```python
from build123d import *

# Parameters (mm, degrees)
F0_R     = 2.179644
F0_R_2   = 5.495
F0_R_3   = 1.811627
F0_R_4   = 2.717522
F1_DEPTH = 3


with BuildPart() as f1:
    # F0 (on Front) → F1 (new body)
    with BuildSketch(Plane.XZ):
        with BuildLine():
            ThreePointArc((4.748624, -43.868074), (19.905522, -31.458489), (38.356329, -38.03854))
            ThreePointArc((38.356329, -38.03854), (48.781106, -31.139926), (36.287612, -31.563568))
            ThreePointArc((36.287612, -31.563568), (34.479775, -16.939453), (26.872979, -4.319244))
            ThreePointArc((26.872979, -4.319244), (26.851679, 10.968683), (15.96134, 21.69816))
            ThreePointArc((15.96134, 21.69816), (22.323636, 32.655587), (20.63084, 45.212594))
            Line((20.63084, 45.212594), (46.282084, 75.748279))
            ThreePointArc((46.282084, 75.748279), (45.843056, 85.044031), (36.784028, 82.913828))
            ThreePointArc((36.784028, 82.913828), (23.791047, 69.810118), (12.145666, 55.495445))
            ThreePointArc((12.145666, 55.495445), (-7.14242, 61.665744), (-26.03866, 54.383233))
            ThreePointArc((-26.03866, 54.383233), (-44.027199, 51.327224), (-32.686998, 37.03294))
            ThreePointArc((-32.686998, 37.03294), (-31.643455, 28.376793), (-26.03866, 21.69816))
            ThreePointArc((-26.03866, 21.69816), (-36.080562, 10.571243), (-37.789793, -4.319244))
            ThreePointArc((-37.789793, -4.319244), (-47.116357, -23.066533), (-44.720202, -43.868074))
            ThreePointArc((-44.720202, -43.868074), (-26.129955, -31.677407), (-7.539708, -43.868074))
            ThreePointArc((-7.539708, -43.868074), (-1.395542, -49.586683), (4.748624, -43.868074))
        make_face()
        with Locations((-39.195588, -22.667399)):
            Circle(F0_R, mode=Mode.SUBTRACT)
        with BuildLine():
            ThreePointArc((2.764325, -43.460141), (-1.413553, -47.586646), (-5.555543, -43.424121))
            ThreePointArc((-5.555543, -43.424121), (-23.64801, -29.816144), (-44.305303, -39.078469))
            ThreePointArc((-44.305303, -39.078469), (-45.548112, -32.328702), (-45.443616, -25.466268))
            ThreePointArc((-45.443616, -25.466268), (-32.535702, -24.254044), (-43.510487, -17.352027))
            ThreePointArc((-43.510487, -17.352027), (-40.221713, -10.719441), (-35.605799, -4.931473))
            ThreePointArc((-35.605799, -4.931473), (-33.578613, 11.124985), (-21.324643, 21.696624))
            ThreePointArc((-21.324643, 21.696624), (-23.830093, 22.711263), (-26.078436, 24.211837))
            Line((-26.078436, 24.211837), (-13.440696, 31.617877))
            ThreePointArc((-13.440696, 31.617877), (-6.255235, 27.617264), (0.930225, 31.617877))
            Line((0.930225, 31.617877), (15.984657, 24.496045))
            ThreePointArc((15.984657, 24.496045), (13.79085, 22.50908), (11.294313, 20.919072))
            ThreePointArc((11.294313, 20.919072), (24.421465, 11.452539), (24.483739, -4.73182))
            ThreePointArc((24.483739, -4.73182), (29.09938, -10.414096), (32.365767, -16.96567))
            ThreePointArc((32.365767, -16.96567), (21.262061, -22.860799), (33.814338, -22.164239))
            ThreePointArc((33.814338, -22.164239), (34.375369, -26.760579), (34.29513, -31.390337))
            ThreePointArc((34.29513, -31.390337), (34.279314, -31.754857), (34.29513, -32.119377))
            ThreePointArc((34.29513, -32.119377), (15.892899, -30.458566), (2.764325, -43.460141))
        make_face(mode=Mode.SUBTRACT)
        with Locations((42.594204, -33.116606)):
            Circle(F0_R_2, mode=Mode.SUBTRACT)
        with Locations((27.461662, -21.133294)):
            Circle(F0_R_3, mode=Mode.SUBTRACT)
        with BuildLine():
            ThreePointArc((-29.585752, 40.232415), (-42.395978, 49.904419), (-26.407067, 51.320147))
            ThreePointArc((-26.407067, 51.320147), (-17.597387, 57.321958), (-7.197797, 59.663057))
            Line((-7.197797, 59.663057), (-7.403995, 44.445188))
            ThreePointArc((-7.403995, 44.445188), (-13.167698, 40.936028), (-14.526525, 34.326333))
            Line((-14.526525, 34.326333), (-28.093472, 26.283829))
            ThreePointArc((-28.093472, 26.283829), (-30.829773, 33.045206), (-29.585752, 40.232415))
        make_face(mode=Mode.SUBTRACT)
        with Locations((-6.255235, 36.070436)):
            Circle(F0_R_4, mode=Mode.SUBTRACT)
        with BuildLine():
            Line((44.843853, 77.145583), (18.220686, 45.452904))
            ThreePointArc((18.220686, 45.452904), (20.692534, 36.023365), (17.751182, 26.729566))
            Line((17.751182, 26.729566), (1.985629, 34.18781))
            ThreePointArc((1.985629, 34.18781), (0.697801, 40.877869), (-5.106476, 44.445188))
            Line((-5.106476, 44.445188), (-5.106476, 59.655479))
            ThreePointArc((-5.106476, 59.655479), (4.312025, 57.645012), (12.521453, 52.609595))
            ThreePointArc((12.521453, 52.609595), (24.714277, 67.842383), (38.436119, 81.713713))
            ThreePointArc((38.436119, 81.713713), (44.55039, 83.512084), (44.843853, 77.145583))
        make_face(mode=Mode.SUBTRACT)
    extrude(amount=F1_DEPTH)


solid = f1.part
```
Part model, mm, in its own coordinate system. Coordinates: 2 decimals unless noted, no trailing zeros. Order: outer loops, then holes, each group sorted by start corner. A loop starts at its lowest first (then second) coordinate and runs counter-clockwise, first axis right, second up. Notation, with made-up numbers: (-40, -34.75) - (9, -34.75) arc R14 cw to (9, -21.75) - close; hole circle Ø8 at (81, -36.5). An arc over 180 degrees is marked (long way). Return JSON: item names as keys, results as strings. Group by question number.
Item 1: Cut at D-D (y = -1.65). State how many separate pieces and enclosed holes the cut face has, plus the area to 3 significant figures.
Item 2: Cut at B-B (x = -17). List the corners of the cut face in (y, z).
Item 3: Pin check, flat tips, straight feed: pin 1 (6.5 mm diameter, centred on x = -6.26, z = 36.07, fed in from -Y); pin 2 (1 mm diameter, centred on y = -1, z = 27, fed in from -X); pin 3 (1 mm diameter, centred on y = -1.5, z = 23, fed in from +X); pin 4 (1.5 mm diameter, centred on y = -2, z = 50.5, fed in from -X). Stop position of each tip, or through.
Item 4: Pull direction Z, two halves, no side cores. Call faces 1 (the face through (44.47, -1.48, 83.57)), 2 (the face through (41.88, -1.48, -27.67)), 3 (the face through (23.96, -1.48, 70)): pulls with the +Z half, pulls with the -Z half, needs draft (parallel to the pull), parting line crosses it, or undercut.
Item 5: Drill centre lines: probe 1 along Z at (x, y) = (26.5, -2.25); probe 2 along X at (y, z) = (-1.65, -36); probe 3 along Z at (x, y) = (-23, -0.55). Where is each one in solid material? Low to high. Write a range as from..to.
Item 6: Cut at C-C (z = -10). List the corners of the cut face in (x, y), plus the area to 3 significant figures.
Item 7: Cut at A-A (z = 47). List the corners of the cut face in (x, y), plus the area to 3 significant figures.
Check values:
{
 "1": {"separate pieces": "1", "enclosed holes": "7", "area": "1,540 mm2"},
 "2": {"outline": "(-3, -33.85) - (0, -33.85) - (0, -31.63) - (-3, -31.63) - close; (-3, 29.53) - (0, 29.53) - (0, 32.86) - (-3, 32.86) - close; (-3, 57.57) - (0, 57.57) - (0, 59.72) - (-3, 59.72) - close"},
 "3": {"pin 1": "stops at y = -3", "pin 2": "stops at x = -31.23", "pin 3": "stops at x = 17.78", "pin 4": "stops at x = -44.49"},
 "4": {"face 1": "undercut", "face 2": "undercut", "face 3": "pulls with the +Z half"},
 "5": {"probe 1": "z = -31.42..-29.4, -27.5..-22.67, -19.6..-14.77, -6.91..11.76, 52.2..55.31, 69.82..72.76", "probe 2": "x = -47.08..-45.04, -41.67..-38.64, -13.62..-10.59, 7.41..10.3, 36.31..37.92, 47.27..48.41", "probe 3": "z = -31.92..-29.9, 21.02..22.31, 26.02..29.3, 54.23..56.67"},
 "6": {"outline": "(-42.13, -3) - (-39.75, -3) - (-39.75, 0) - (-42.13, 0) - close; (28.83, -3) - (31.2, -3) - (31.2, 0) - (28.83, 0) - close", "area": "14.3 mm2"},
 "7": {"outline": "(-44.72, -3) - (-42.71, -3) - (-42.71, 0) - (-44.72, 0) - close; (-7.37, -3) - (-5.11, -3) - (-5.11, 0) - (-7.37, 0) - close; (19.52, -3) - (22.13, -3) - (22.13, 0) - (19.52, 0) - close", "area": "20.6 mm2"}
}
